The model under review builds one solid part; all positions refer to its coordinate system, in mm. Face numbers are marked on the shaded views. A direction names the side the tool comes from. Round coordinates to 2 decimals unless told otherwise and drop trailing zeros. Write each loop counter-clockwise with the first axis right and the second up, starting at its lowest first coordinate (ties: lowest second). Pieces come first, ordered by that corner, then holes. Notation, with made-up numbers: M 36.5,14.5 L 90.5,14.5 A18 cw 90.5,30.5 Z; hole C 30.5,48.25 d11. An arc over 180 degrees is marked long. Write item = value, one per line. Start each with the question number.
Item 1: Take a section at B-B, the plane z = 17. Give the boundary of the cut face in (x, y), plus the area to 4 significant figures.
Item 2: To check wall thickness, follow line 1 along X through (y, z) = (10, 4.5); line 2 along Z through (x, y) = (14.75, 20); line 3 along Y through (x, z) = (1, 12.5). State the ranges of each line that lie inside material, in increasing order.
Item 3: The part is to be moulded in two halves that separate along Z. For the marked faces 1, 2, 3 and 4, say which applies: +Z half, -Z half, draft (parallel to the pull), parting line (faces both ways), or undercut.
Item 4: Take a section at D-D, the plane y = 19.5. Give the boundary of the cut face in (x, z), plus the area to 4 significant figures.
Item 5: Take a section at A-A, the plane y = 7. Give the boundary of the cut face in (x, z), plus the area to 3 significant figures.
Item 6: Tool access review of the marked faces 5, 6, 7 and 8: name each direction out of +Z, -Z, +X, -X, +Y, -Y from which nothing blocks a thin tool from reaching the whole face with its end or side.
Item 7: Take a section at C-C, the plane x = 15.25. Give the boundary of the cut face in (y, z).
Item 8: For pin 1 Ø2.5 at (x, z) = (10.5, 15.5) entering from +Y; pin 2 Ø12 at (y, z) = (20, 22) entering from -X; pin 3 Ø2 at (x, z) = (5.5, 19.5) entering from +Y, all flat-tipped, find the tip position at first contact; note any pin that passes through.
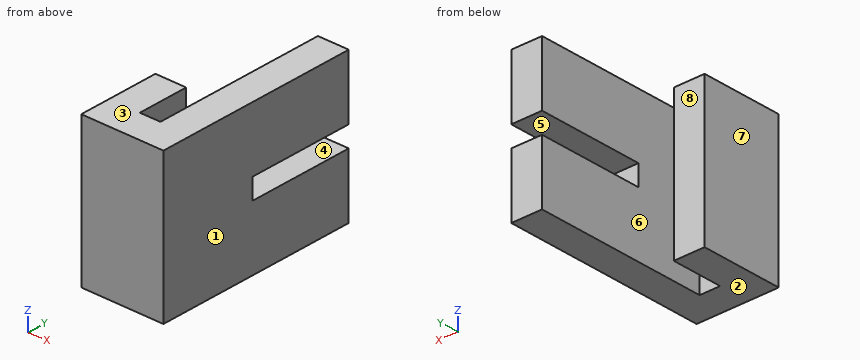
Autodesk Fusion 360 part; units mm, degrees
sketch "Sketch1" plane through (0, 0, 0) normal (0, 0, 1) x (1, 0, 0)
  line L0 (0, 0) -> (7.5, 0)
  line L1 (7.5, 0) -> (7.5, 12.5)
  line L2 (7.5, 12.5) -> (0, 12.5)
  line L3 (0, 12.5) -> (0, 0)
  line L4 (0, 0) -> (12.5, 0)
  line L5 (12.5, 0) -> (12.5, -7.5)
  line L6 (12.5, -7.5) -> (0, -7.5)
  line L7 (0, -7.5) -> (0, 0)
  line L8 (12.5, -7.5) -> (20, -7.5)
  line L9 (20, -7.5) -> (20, 42.5)
  line L10 (20, 42.5) -> (12.5, 42.5)
  line L11 (12.5, 42.5) -> (12.5, -7.5)
  dimension "d1" = 12.5
  dimension "d2" = 50
  dimension "d3" = 7.5
  dimension "d4" = 7.5
  dimension "d5" = 7.5
  dimension "d6" = 12.5
extrude "Extrude1" add sketch "Sketch1" along normal blind 36
sketch "Sketch2" plane through (20, 0, 0) normal (1, 0, 0) x (0, 1, 0)
  line L0 (-7.5, 36) -> (42.5, 36)
  line L1 (42.5, 36) -> (42.5, 0)
  line L2 (42.5, 0) -> (-7.5, 0)
  line L3 (-7.5, 0) -> (-7.5, 36)
  line L4 (42.5, 20.5) -> (16.5, 20.5)
  line L5 (16.5, 20.5) -> (16.5, 15.5)
  line L6 (16.5, 15.5) -> (42.5, 15.5)
  line L7 (42.5, 15.5) -> (42.5, 20.5)
  dimension "d13" = 15.5
  dimension "d14" = 15.5
  dimension "d16" = 24
  dimension "d17" = 50
  dimension "d19" = 36
  dimension "d21" = 5
extrude "Extrude2" cut sketch "Sketch2" along normal through all and the other way through all contours L1 L4 L5 L6 L7
Response values:
q1.outline = M 0,-7.5 L 20,-7.5 L 20,16.5 L 12.5,16.5 L 12.5,0 L 7.5,0 L 7.5,12.5 L 0,12.5 Z
q1.area = 367.5 mm2
q2.line_1 = 0 to 7.5, 12.5 to 20
q2.line_2 = 0 to 15.5, 20.5 to 36
q2.line_3 = -7.5 to 12.5
q3.face_1 = draft
q3.face_2 = -Z half
q3.face_3 = +Z half
q3.face_4 = undercut
q4.outline = M 12.5,0 L 20,0 L 20,15.5 L 12.5,15.5 Z; M 12.5,20.5 L 20,20.5 L 20,36 L 12.5,36 Z
q4.area = 232.5 mm2
q5.outline = M 0,0 L 7.5,0 L 7.5,36 L 0,36 Z; M 12.5,0 L 20,0 L 20,36 L 12.5,36 Z
q5.area = 540 mm2
q6.face_5 = +X, -X, +Y
q6.face_6 = +Z, -Z, +Y
q6.face_7 = +Z, -Z, -X, +Y, -Y
q6.face_8 = +Z, -Z, -X, +Y
q7.outline = M -7.5,0 L 42.5,0 L 42.5,15.5 L 16.5,15.5 L 16.5,20.5 L 42.5,20.5 L 42.5,36 L -7.5,36 Z
q8.pin_1 = 0
q8.pin_2 = 12.5
q8.pin_3 = 12.5
